Here's the drawing with two shaded views (mm, measured from the low corner). I have some questions. A direction names the side the tool comes from. Round coordinates to 2 decimals unless told otherwise and drop trailing zeros. Loops run counter-clockwise (first coordinate to the right, second up) from the corner with the lowest first, then second, coordinate; pieces in that order, holes last.
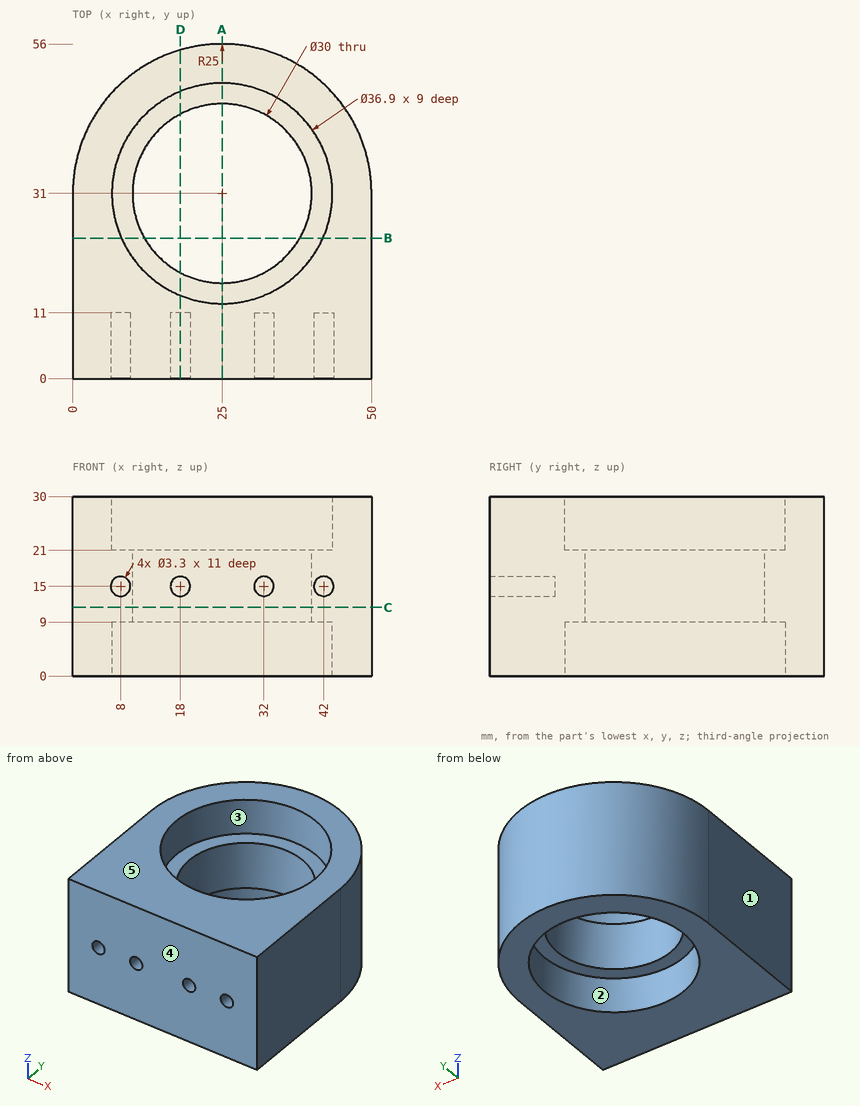
(1) If we section it at A-A, the plane x = 25: List the corners of the cut face in (y, z) for me, then the cut area to 3 significant figures.
Worked answers:
outline: (0, 0) - (12.55, 0) - (12.55, 9) - (16, 9) - (16, 21) - (12.55, 21) - (12.55, 30) - (0, 30) - close; (46, 9) - (49.45, 9) - (49.45, 0) - (56, 0) - (56, 30) - (49.45, 30) - (49.45, 21) - (46, 21) - close
area: 656 mm2
(2) For the marked faces 1 and 2, which set-ups out of +Z, -Z, +X, -X, +Y, -Y let a thin tool reach every point of the face, with its end or its side?
Worked answers:
face 1: +Z, -Z, -X, +Y, -Y
face 2: -Z
(3) Will these pins go through, and if not, where does the flat tip stop? P1, Ø1, axis at x = 22.5, z = 3.5, coming from the +Y side; P2, Ø24, axis at x = 25, y = 31, coming from the -Z side; P3, Ø1, axis at x = 43, z = 15, coming from the -Y side; P4, Ø8, axis at x = 16, y = 22, coming from the -Z side.
Worked answers:
P1: stops at y = 55.92
P2: passes through
P3: stops at y = 11
P4: stops at z = 9
(4) If we section it at C-C, the plane z = 11.5: List the corners of the cut face in (x, y) for me.
Worked answers:
outline: (0, 0) - (50, 0) - (50, 31) arc R25 ccw to (0, 31) - close; hole circle Ø30 at (25, 31)
(5) If we section it at B-B, the plane y = 23.5: List the corners of the cut face in (x, z) for me.
Worked answers:
outline: (0, 0) - (8.14, 0) - (8.14, 9) - (12.01, 9) - (12.01, 21) - (8.14, 21) - (8.14, 30) - (0, 30) - close; (37.99, 9) - (41.86, 9) - (41.86, 0) - (50, 0) - (50, 30) - (41.86, 30) - (41.86, 21) - (37.99, 21) - close
(6) If I drill on line 1 (X direction, y = 6.5, z = 15); line 2 (Y direction, x = 25, z = 24.5); line 3 (Y direction, x = 25.5, z = 10.5) (3 decimals), over which ranges is the centre line in solid material (lowest first)?
Worked answers:
line 1: x = 0 to 6.35, 9.65 to 16.35, 19.65 to 30.35, 33.65 to 40.35, 43.65 to 50
line 2: y = 0 to 12.55, 49.45 to 56
line 3: y = 0 to 16.008, 45.992 to 55.995
(7) If we mould it in two halves opening along Y, with no side actions, what happens to the marked faces 3, 4 and 5? For each: released by +Y, released by -Y, zero draft, split by the parting line, or undercut.
Worked answers:
face 3: undercut
face 4: released by -Y
face 5: zero draft
(8) If we section it at D-D, the plane x = 18: List the corners of the cut face in (y, z) for me, then the cut area to 3 significant figures.
Worked answers:
outline: (0, 0) - (13.93, 0) - (13.93, 9) - (17.73, 9) - (17.73, 21) - (13.93, 21) - (13.93, 30) - (0, 30) - (0, 16.65) - (11, 16.65) - (11, 13.35) - (0, 13.35) - close; (44.27, 9) - (48.07, 9) - (48.07, 0) - (55, 0) - (55, 30) - (48.07, 30) - (48.07, 21) - (44.27, 21) - close
area: 681 mm2
